from build123d import *

# Parameters (mm, degrees)
BOSS_EXTRUDE1_DEPTH            = 2.54
F_7_16_0_4375_DIAMETER_HOLE1_D = 11.1125
F_8_CLEARANCE_HOLE2_D          = 4.4958
F_10_CLEARANCE_HOLE2_D         = 5.1054


with BuildPart() as part:
    # Sketch1 → Boss-Extrude1 (new body)
    with BuildSketch(Plane(origin=(0, 0, 0), x_dir=(0, 0, -1), z_dir=(1, 0, 0))):
        with BuildLine():
            Line((-19.314481315, -36.508827357), (37.835518685, -38.096327357))
            ThreePointArc((37.835518685, -38.096327357), (43.508241138, -36.415698489), (47.094324235, -31.709925286))
            ThreePointArc((47.094324235, -31.709925286), (49.666291071, -27.372500374), (53.723446842, -24.377879309))
            ThreePointArc((53.723446842, -24.377879309), (56.748764885, -22.739945951), (59.555317673, -20.750313723))
            ThreePointArc((59.555317673, -20.750313723), (70.190449205, -13.830311686), (81.989075544, -9.162885478))
            ThreePointArc((81.989075544, -9.162885478), (88.904940009, -0.38440552), (82.719582069, 8.923238587))
            ThreePointArc((82.719582069, 8.923238587), (71.335814009, 14.527011927), (61.293419407, 22.282188362))
            ThreePointArc((61.293419407, 22.282188362), (57.164774633, 25.524177799), (52.512741108, 27.956211363))
            ThreePointArc((52.512741108, 27.956211363), (48.982518098, 30.139520785), (46.344839733, 33.344511796))
            ThreePointArc((46.344839733, 33.344511796), (42.509528769, 37.017847922), (37.303469713, 38.066636556))
            Line((37.303469713, 38.066636556), (18.518979809, 36.490257704))
            ThreePointArc((18.518979809, 36.490257704), (14.772389284, 34.855531703), (12.798400928, 31.276056933))
            ThreePointArc((12.798400928, 31.276056933), (12.18571912, 18.160305029), (14.955046072, 5.325619398))
            ThreePointArc((14.955046072, 5.325619398), (12.972274915, -9.150721749), (0, -15.875))
            ThreePointArc((0, -15.875), (-10.349023893, -16.30546329), (-20.626551724, -17.59387931))
            ThreePointArc((-20.626551724, -17.59387931), (-28.552166362, -27.646635371), (-19.314481315, -36.508827357))
        make_face()
        with BuildLine():
            Line((28.956, 7.874), (28.956, -4.826))
            ThreePointArc((28.956, -4.826), (32.675743879, -13.806256121), (41.656, -17.526))
            ThreePointArc((41.656, -17.526), (60.706, 1.524), (41.656, 20.574))
            ThreePointArc((41.656, 20.574), (32.675743879, 16.854256121), (28.956, 7.874))
        make_face(mode=Mode.SUBTRACT)
    extrude(amount=BOSS_EXTRUDE1_DEPTH)

    # 7/16 (0.4375) Diameter Hole1 (through all)
    with Locations(Plane(origin=(2.54, 0, 0), x_dir=(0, 0, -1), z_dir=(1, 0, 0))):
        with Locations((19.05, -26.9875)):
            Hole(F_7_16_0_4375_DIAMETER_HOLE1_D / 2)

    # #8 Clearance Hole2 (through all)
    with Locations(Plane(origin=(2.54, 0, 0), x_dir=(0, 0, -1), z_dir=(1, 0, 0))):
        with Locations((38.1, -28.575), (79.3877, 0), (38.1, 28.575)):
            Hole(F_8_CLEARANCE_HOLE2_D / 2)

    # #10 Clearance Hole2 (through all)
    with Locations(Plane(origin=(2.54, 0, 0), x_dir=(0, 0, -1), z_dir=(1, 0, 0))):
        with Locations((-19.05, -26.9875), (19.05, 30.1625)):
            Hole(F_10_CLEARANCE_HOLE2_D / 2)


solid = part.part
Check sheet for the modelled part. Datum: model origin and axes. Units: mm. A direction names the side the tool comes from. Coordinates: 2 decimals unless noted, no trailing zeros. Write each loop counter-clockwise with the first axis right and the second up, starting at its lowest first coordinate (ties: lowest second). Pieces come first, ordered by that corner, then holes.
Item 1: Scan lines: probe 1 along Z at (x, y) = (1.5, -25); probe 2 along Z at (x, y) = (1.4, 30); probe 3 along Y at (x, z) = (0.95, -38.1). Record each from-to range of solid material in increasing order.
Numbers:
probe 1: z = -52.55 to -24.24, -13.86 to 17.45, 20.65 to 28.37
probe 2: z = -49.14 to -39.84, -36.36 to -21.6, -16.5 to -12.59
probe 3: y = -38.1 to -30.82, -26.33 to -17.02, 20.07 to 26.33, 30.82 to 38.1
Item 2: Mould release check, pull along Z, two halves, no side actions. Record for faces 1 (the face through (1.252, -22.765, -56.708)), 2 (the face through (1.25, -8.98, -13.09)), 3 (the face through (1.3, 1.1, -60.7)): released by +Z, released by -Z, zero draft, split by the parting line, or undercut.
Numbers:
face 1: released by -Z
face 2: released by +Z
face 3: undercut
Item 3: Cross-section at B-B on x = 1.9. Count the separate pieces of the cut face and the enclosed holes in it, then the cut area to 3 significant figures.
Numbers:
separate pieces: 1
enclosed holes: 7
area: 3,580 mm2
Item 4: Access from +Z, -Z, +X, -X, +Y, -Y to the whole of each face (thin tool, end or side, straight path). Record for faces 4 (the face through (1.25, -13.71, -32.58)), 5 (the face through (1.25, 18.34, -12.17)).
Numbers:
face 4: +X, -X
face 5: +Z, +X, -X
Item 5: Cross-section at A-A on y = 0. Record the boundary of the cut face in (x, z) (3 decimals).
Numbers:
outline: (0, -88.913) - (2.54, -88.913) - (2.54, -81.636) - (0, -81.636) - close; (0, -77.14) - (2.54, -77.14) - (2.54, -60.645) - (0, -60.645) - close; (0, -28.956) - (2.54, -28.956) - (2.54, -15.875) - (0, -15.875) - close
Item 6: Depth check by flat-ended pin: pin 1 Ø10 at (y, z) = (20, -64.5) entering from -X; pin 2 Ø1 at (x, y) = (2, 13) entering from -Z; pin 3 Ø10 at (y, z) = (-24, -67.5) entering from +X. Enter the tip coordinate at first touch or a pass-through.
Numbers:
pin 1: stops at x = 0
pin 2: stops at z = -74.83
pin 3: passes through
